Can you work these out from the drawing? Everything is in mm from the part's minimum corner. Coordinates: 2 decimals unless noted, no trailing zeros. Order: outer loops, then holes, each group sorted by start corner. A loop starts at its lowest first (then second) coordinate and runs counter-clockwise, first axis right, second up. Notation, with made-up numbers: (31, -9) -> (82, -9) arc R20 ccw to (82, 8) -> close; hole circle Ø10 at (-33.5, 62.25). An arc over 180 degrees is marked (long way). Put each result on its own line as item: value. Start each with the question number.
Q1. If we section it at C-C (z = 6.75): Please give me the cut outline in (x, y).
Q2. Please list where these lines run through material, in increasing order: line 1 along Y through (x, z) = (294, 3.25); line 2 along X through (y, z) = (190, 3).
Q3. If we section it at A-A (y = 125.5): Please give me the cut outline in (x, z).
Q4. If we section it at B-B (x = 256): Please give me the cut outline in (y, z).
Q5. Will these pins go through, and if not, where does the flat tip stop? pin 1 (11 mm diameter, centred on y = 78.5, z = 7.5, fed in from -X); pin 2 (5 mm diameter, centred on x = 196, z = 15.5, fed in from -Y); pin 3 (11 mm diameter, centred on y = 54.5, z = 9, fed in from +X).
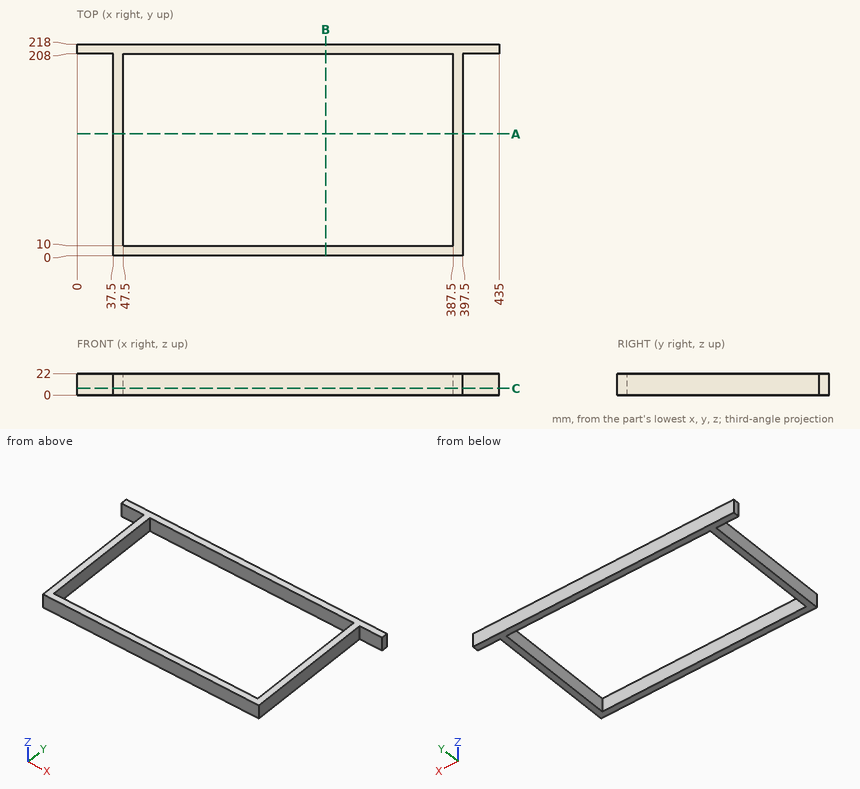
The answers:
1. outline: (0, 208) -> (37.5, 208) -> (37.5, 0) -> (397.5, 0) -> (397.5, 208) -> (435, 208) -> (435, 218) -> (0, 218) -> close; hole (47.5, 10) -> (387.5, 10) -> (387.5, 208) -> (47.5, 208) -> close
2. line 1: 0 to 10, 208 to 218
2. line 2: 37.5 to 47.5, 387.5 to 397.5
3. outline: (37.5, 0) -> (47.5, 0) -> (47.5, 22) -> (37.5, 22) -> close; (387.5, 0) -> (397.5, 0) -> (397.5, 22) -> (387.5, 22) -> close
4. outline: (0, 0) -> (10, 0) -> (10, 22) -> (0, 22) -> close; (208, 0) -> (218, 0) -> (218, 22) -> (208, 22) -> close
5. pin 1: x = 37.5
5. pin 2: y = 0
5. pin 3: x = 397.5
